Design review of the part built by this model. Coordinates are the model's own, in mm. Give positions to 0.01 mm unless a question says otherwise; leave off trailing zeros. Loops run counter-clockwise (first coordinate to the right, second up) from the corner with the lowest first, then second, coordinate; pieces in that order, holes last. Notation, with made-up numbers: (79.25, 78.25) -> (134.25, 78.25) arc R25 cw to (134.25, 105.25) -> close; hole circle Ø10 at (-32.5, 53). An arc over 180 degrees is marked (long way). Use a Markdown table: item, result. Add a question column.
1. For pin 1 Ø2.5 at (x, y) = (100.5, 2.5) entering from -Z; pin 2 Ø2.5 at (x, y) = (103.5, 2) entering from +Z, all flat-tipped, find the tip position at first contact; note any pin that passes through.
2. Add section A-A (z = 183.5). State the section outline as (x, y) points, and give its area (3 significant figures).
3. Add section C-C (x = 109.5). State the section outline as (y, z) points.
4. Add section B-B (y = 3.7). State the section outline as (x, z) points, and give its area (3 significant figures).
5. To check wall thickness, follow line 1 (X direction, y = 3.9, z = 163.5); line 2 (Z direction, x = 84.5, y = 2.85). State the ranges of each line that lie inside material, in increasing order.
Autodesk Inventor part; units mm, degrees
ref_plane "YZ Plane" through (0, 0, 0) normal (1, 0, 0) x (0, 1, 0)
ref_plane "XZ Plane" through (0, 0, 0) normal (0, 1, 0) x (-1, 0, 0)
ref_plane "XY Plane" through (0, 0, 0) normal (0, 0, 1) x (1, 0, 0)
sketch "Sketch1" plane through (0, 0, 0) normal (0, 1, 0) x (-1, 0, 0)
  line L0 (171.4161, 216.9837) -> (-425.4839, 216.9837)
  line L1 (-425.4839, 216.9837) -> (-425.4839, -100.5163)
  line L2 (-425.4839, -100.5163) -> (171.4161, -100.5163)
  line L3 (171.4161, -100.5163) -> (171.4161, 216.9837)
  point P0 (0, 0)
  dimension "d0" = 317.5
  dimension "d1" = 596.9
extrude "Extrusion1" add sketch "Sketch1" along normal blind 4.7625
sketch "Sketch2" plane through (0, 4.7625, 0) normal (0, 1, 0) x (1, 0, 0)
  line L0 (57.1839, 30.6663) -> (196.8839, 30.6663)
  line L1 (196.8839, 30.6663) -> (196.8839, 100.5163)
  line L2 (196.8839, 100.5163) -> (57.1839, 100.5163)
  line L3 (57.1839, 100.5163) -> (57.1839, 30.6663)
  line L4 (57.1839, -147.1337) -> (196.8839, -147.1337)
  line L5 (196.8839, -147.1337) -> (196.8839, -216.9837)
  line L6 (196.8839, -216.9837) -> (57.1839, -216.9837)
  line L7 (57.1839, -216.9837) -> (57.1839, -147.1337)
  line L8 (425.4839, -216.9837) -> (425.4839, 100.5163)
  line L9 (-171.4161, 100.5163) -> (-171.4161, -216.9837)
  line L10 (-171.4161, -216.9837) -> (425.4839, -216.9837)
  line L11 (425.4839, 100.5163) -> (-171.4161, 100.5163)
  point P0 (0, 0)
  dimension "d4" = 0
  dimension "d5" = 228.6
  dimension "d6" = 0
  dimension "d7" = 228.6
  dimension "d8" = 0
  dimension "d9" = 0
  dimension "d10" = 69.85
  dimension "d11" = 69.85
extrude "Extrusion2" cut sketch "Sketch2" along normal mid plane 25.4 contours L3 L2 L1 L0 | L7 L4 L5 L6
sketch "Sketch3" plane through (0, 4.7625, 0) normal (0, 1, 0) x (1, 0, 0)
  line L0 (-203.1439, 127.0873) -> (472.3707, 127.0873)
  line L1 (472.3707, 127.0873) -> (472.3707, 90.9913)
  line L2 (472.3707, 90.9913) -> (-203.1439, 90.9913)
  line L3 (-203.1439, 90.9913) -> (-203.1439, 127.0873)
  line L4 (463.6684, -207.4587) -> (-190.0904, -207.4587)
  line L5 (-190.0904, -207.4587) -> (-190.0904, -244.0242)
  line L6 (-190.0904, -244.0242) -> (463.6684, -244.0242)
  line L7 (463.6684, -244.0242) -> (463.6684, -207.4587)
  line L8 (425.4839, 100.5163) -> (196.8839, 100.5163)
  line L9 (196.8839, -216.9837) -> (425.4839, -216.9837)
  point P0 (0, 0)
  dimension "d14" = 9.525
  dimension "d15" = 9.525
extrude "Extrusion3" cut sketch "Sketch3" against normal blind 25.4
properties part number "EBoard" material "Polycarbonate, Clear"
Taken from the geometry:
| question | item | result |
|---|---|---|
| 1 | pin 1 | stops at z = -30.67 |
| 1 | pin 2 | stops at z = 147.13 |
| 2 | outline | (-171.42, 0) -> (57.18, 0) -> (57.18, 4.76) -> (-171.42, 4.76) -> close; (196.88, 0) -> (425.48, 0) -> (425.48, 4.76) -> (196.88, 4.76) -> close |
| 2 | area | 2,180 mm^2 |
| 3 | outline | (0, -30.67) -> (4.76, -30.67) -> (4.76, 147.13) -> (0, 147.13) -> close |
| 4 | outline | (-171.42, -90.99) -> (57.18, -90.99) -> (57.18, -30.67) -> (196.88, -30.67) -> (196.88, -90.99) -> (425.48, -90.99) -> (425.48, 207.46) -> (196.88, 207.46) -> (196.88, 147.13) -> (57.18, 147.13) -> (57.18, 207.46) -> (-171.42, 207.46) -> close |
| 4 | area | 161,000 mm^2 |
| 5 | line 1 | x = -171.42 to 57.18, 196.88 to 425.48 |
| 5 | line 2 | z = -30.67 to 147.13 |
